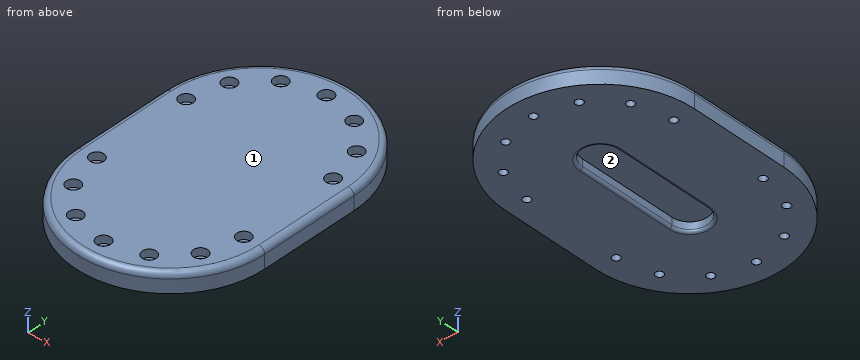
from build123d import *

# Parameters (mm, degrees)
BOSS_EXTRUDE1_DEPTH        = 12.5
CUT_EXTRUDE1_DEPTH         = 6.25
FILLET1_R                  = 1.75
FILLET2_R                  = 3.75
HOLE1_D                    = 5
HOLE1_DEPTH                = 30
HOLE1_CBORE_D              = 9
HOLE1_CBORE_DEPTH          = 5
CIRPATTERN1_COUNT          = 7
CIRPATTERN1_ANGLE          = 180
MIRROR1_COPY_1_D           = 5
MIRROR1_COPY_1_DEPTH       = 30
MIRROR1_COPY_1_CBORE_D     = 9
MIRROR1_COPY_1_CBORE_DEPTH = 5
MIRROR1_COPY_2_D           = 5
MIRROR1_COPY_2_DEPTH       = 30
MIRROR1_COPY_2_CBORE_D     = 9
MIRROR1_COPY_2_CBORE_DEPTH = 5
MIRROR1_COPY_3_D           = 5
MIRROR1_COPY_3_DEPTH       = 30
MIRROR1_COPY_3_CBORE_D     = 9
MIRROR1_COPY_3_CBORE_DEPTH = 5
MIRROR1_COPY_4_D           = 5
MIRROR1_COPY_4_DEPTH       = 30
MIRROR1_COPY_4_CBORE_D     = 9
MIRROR1_COPY_4_CBORE_DEPTH = 5
MIRROR1_COPY_5_D           = 5
MIRROR1_COPY_5_DEPTH       = 30
MIRROR1_COPY_5_CBORE_D     = 9
MIRROR1_COPY_5_CBORE_DEPTH = 5
MIRROR1_COPY_6_D           = 5
MIRROR1_COPY_6_DEPTH       = 30
MIRROR1_COPY_6_CBORE_D     = 9
MIRROR1_COPY_6_CBORE_DEPTH = 5


with BuildPart() as part:
    # Sketch1 → Boss-Extrude1 (new body)
    with BuildSketch(Plane.XY):
        with BuildLine():
            Line((61, 31.75), (61, -31.75))
            ThreePointArc((61, -31.75), (0, -92.75), (-61, -31.75))
            Line((-61, -31.75), (-61, 31.75))
            ThreePointArc((-61, 31.75), (0, 92.75), (61, 31.75))
        make_face()
    extrude(amount=BOSS_EXTRUDE1_DEPTH)

    # Sketch1<3> → Cut-Extrude1 (cut)
    with BuildSketch(Plane.XY):
        with BuildLine():
            Line((-11.5, 31.75), (-11.5, -31.75))
            ThreePointArc((-11.5, -31.75), (0, -43.25), (11.5, -31.75))
            Line((11.5, -31.75), (11.5, 31.75))
            ThreePointArc((11.5, 31.75), (0, 43.25), (-11.5, 31.75))
        make_face()
    extrude(amount=CUT_EXTRUDE1_DEPTH, mode=Mode.SUBTRACT)

    # Fillet1
    fillet1_edges = [part.edges().sort_by_distance(p)[0] for p in [
        (-11.5, 0, 0),
        (0, -43.25, 0),
        (0, 43.25, 0),
        (11.5, 0, 0),
    ]]
    fillet(fillet1_edges, radius=FILLET1_R)

    # Fillet2
    fillet2_edges = [part.edges().sort_by_distance(p)[0] for p in [
        (0, -92.75, 12.5),
        (61, 0, 12.5),
        (0, 92.75, 12.5),
        (-61, 0, 12.5),
    ]]
    fillet(fillet2_edges, radius=FILLET2_R)

    # Hole1
    with Locations(Plane.XY.offset(12.5)):
        with Locations((-47.5, 31.75)):
            hole1 = CounterBoreHole(HOLE1_D / 2, HOLE1_CBORE_D / 2, HOLE1_CBORE_DEPTH, depth=HOLE1_DEPTH)

    # CirPattern1: Hole1 ×7 about axis
    cirpattern1_axis = Axis((0, 31.75, 0), (0, 0, -1))
    for i in range(1, CIRPATTERN1_COUNT):
        add(hole1.rotate(cirpattern1_axis, i * CIRPATTERN1_ANGLE / (CIRPATTERN1_COUNT - 1)), mode=Mode.SUBTRACT)

    # Mirror1: Hole1 across plane
    add(hole1.mirror(Plane.ZX), mode=Mode.SUBTRACT)

    # Mirror1 copy 1
    with Locations(Plane(origin=(-15.875, -4.25369343, 12.5), x_dir=(0.866025404, 0.5, 0), z_dir=(0, 0, 1))):
        with Locations((-47.5, -31.75)):
            CounterBoreHole(MIRROR1_COPY_1_D / 2, MIRROR1_COPY_1_CBORE_D / 2, MIRROR1_COPY_1_CBORE_DEPTH, depth=MIRROR1_COPY_1_DEPTH)

    # Mirror1 copy 2
    with Locations(Plane(origin=(-27.49630657, -15.875, 12.5), x_dir=(0.5, 0.866025404, 0), z_dir=(0, 0, 1))):
        with Locations((-47.5, -31.75)):
            CounterBoreHole(MIRROR1_COPY_2_D / 2, MIRROR1_COPY_2_CBORE_D / 2, MIRROR1_COPY_2_CBORE_DEPTH, depth=MIRROR1_COPY_2_DEPTH)

    # Mirror1 copy 3
    with Locations(Plane(origin=(-31.75, -31.75, 12.5), x_dir=(0, 1, 0), z_dir=(0, 0, 1))):
        with Locations((-47.5, -31.75)):
            CounterBoreHole(MIRROR1_COPY_3_D / 2, MIRROR1_COPY_3_CBORE_D / 2, MIRROR1_COPY_3_CBORE_DEPTH, depth=MIRROR1_COPY_3_DEPTH)

    # Mirror1 copy 4
    with Locations(Plane(origin=(-27.49630657, -47.625, 12.5), x_dir=(-0.5, 0.866025404, 0), z_dir=(0, 0, 1))):
        with Locations((-47.5, -31.75)):
            CounterBoreHole(MIRROR1_COPY_4_D / 2, MIRROR1_COPY_4_CBORE_D / 2, MIRROR1_COPY_4_CBORE_DEPTH, depth=MIRROR1_COPY_4_DEPTH)

    # Mirror1 copy 5
    with Locations(Plane(origin=(-15.875, -59.24630657, 12.5), x_dir=(-0.866025404, 0.5, 0), z_dir=(0, 0, 1))):
        with Locations((-47.5, -31.75)):
            CounterBoreHole(MIRROR1_COPY_5_D / 2, MIRROR1_COPY_5_CBORE_D / 2, MIRROR1_COPY_5_CBORE_DEPTH, depth=MIRROR1_COPY_5_DEPTH)

    # Mirror1 copy 6
    with Locations(Plane(origin=(0, -63.5, 12.5), x_dir=(-1, 0, 0), z_dir=(0, 0, 1))):
        with Locations((-47.5, -31.75)):
            CounterBoreHole(MIRROR1_COPY_6_D / 2, MIRROR1_COPY_6_CBORE_D / 2, MIRROR1_COPY_6_CBORE_DEPTH, depth=MIRROR1_COPY_6_DEPTH)


solid = part.part
The listing builds one solid part. Answer for the finished solid, in the listing's coordinates (mm). Face numbers are marked on the shaded views. Coordinates: 2 decimals unless noted, no trailing zeros. Write each loop counter-clockwise with the first axis right and the second up, starting at its lowest first coordinate (ties: lowest second). Pieces come first, ordered by that corner, then holes. Notation, with made-up numbers: M 11,43 L 41,43 A12 cw 41,64 Z; hole C 25,-33 d6. An arc over 180 degrees is marked long. Write each question's results on one line, items separated by ' | '.
Item 1: The part is cut by section A-A on x = 0. Determine the outline of the cut face in (y, z), and give its area (3 significant figures).
Answer below:
outline: M -92.75,0 L -81.75,0 L -81.75,7.5 L -83.75,7.5 L -83.75,12.5 L -89,12.5 A3.75 ccw -92.75,8.75 Z; M -76.75,0 L -45,0 A1.75 ccw -43.25,1.75 L -43.25,6.25 L 43.25,6.25 L 43.25,1.75 A1.75 ccw 45,0 L 76.75,0 L 76.75,7.5 L 74.75,7.5 L 74.75,12.5 L -74.75,12.5 L -74.75,7.5 L -76.75,7.5 Z; M 81.75,0 L 92.75,0 L 92.75,8.75 A3.75 ccw 89,12.5 L 83.75,12.5 L 83.75,7.5 L 81.75,7.5 Z | area: 1,610 mm2
Item 2: For a pull along Y with two mould halves and no side action, classify the marked faces 1 and 2 as released by +Y, released by -Y, zero draft, split by the parting line, or undercut.
Answer below:
face 1: zero draft | face 2: undercut
Item 3: The part is cut by section C-C on x = -47.5. State how many separate pieces and enclosed holes the cut face has, and give its area (3 significant figures).
Answer below:
separate pieces: 3 | enclosed holes: 0 | area: 1,580 mm2
Item 4: Given P1, Ø5, axis at x = -12.5, z = 11, coming from the +Y side; P2, Ø1.5, axis at x = -19.5, z = 9, coming from the +Y side; P3, Ø18.5, axis at x = -3, y = 0.5, coming from the -Z side, each flat-ended and moving along its own axis, determine where each tip first touches the part or whether it passes through.
Answer below:
P1: y = 91.77 | P2: y = 89.79 | P3: z = 0.31
Item 5: The part is cut by section B-B on y = 9. Determine the outline of the cut face in (x, z).
Answer below:
outline: M -61,0 L -13.25,0 A1.75 ccw -11.5,1.75 L -11.5,6.25 L 11.5,6.25 L 11.5,1.75 A1.75 ccw 13.25,0 L 61,0 L 61,8.75 A3.75 ccw 57.25,12.5 L -57.25,12.5 A3.75 ccw -61,8.75 Z
Item 6: Consider probe 1 along Y at (x, z) = (-37, 10); probe 2 along X at (y, z) = (-70.5, 11.25); probe 3 along X at (y, z) = (-55.5, 3.5). Determine where each line is inside the solid, lowest interval first. Write a range as [from, to].
Answer below:
probe 1: [-79.98, -57.27], [-53.73, 53.73], [57.27, 79.98] | probe 2: [-45.87, -27.57], [-19.93, 19.93], [27.57, 45.87] | probe 3: [-56.19, -43.64], [-38.64, 38.64], [43.64, 56.19]
